Geometry check sheet. Reference: the model listing, model coordinates, mm. Face numbers are marked on the shaded views. A direction names the side the tool comes from. Round coordinates to 2 decimals unless told otherwise and drop trailing zeros. Order: outer loops, then holes, each group sorted by start corner. A loop starts at its lowest first (then second) coordinate and runs counter-clockwise, first axis right, second up.
```python
from build123d import *

# Parameters (mm, degrees)
EXTRUDE_1_DEPTH                 = 206
SKETCH_3_W                      = 252
SKETCH_3_H                      = 252
CUT_EXTRUDE_1_DEPTH             = 123.6
SKETCH_5_W                      = 210
SKETCH_5_H                      = 210
CUT_EXTRUDE_5_DEPTH             = 20.6
SHELL_9_T                       = -5
SKETCH_6_R                      = 50
CUT_EXTRUDE_6_DEPTH             = 455.80065963
RIB_START                       = -5
RIB_1_DEPTH                     = 10
PATTERN_CIRCULAR_1_COUNT        = 4
PATTERN_START                   = -5
PATTERN_CIRCULAR_1_COPY_1_DEPTH = 10
PATTERN_CIRCULAR_1_COPY_2_DEPTH = 10
PATTERN_CIRCULAR_1_COPY_3_DEPTH = 10


# Read off the part's stored shape, not the designer's step: the rib step
with BuildPart() as part:
    # Sketch 1 → Extrude 1 (new body)
    with BuildSketch(Plane(origin=(0, 0, 0), x_dir=(1, 0, 0), z_dir=(0, 1, 0))):
        Polygon((-305, 183), (-183, 305), (183, 305), (305, 183), (305, -183), (183, -305), (-183, -305), (-305, -183), align=None)
    extrude(amount=EXTRUDE_1_DEPTH)

    # Sketch 3 → Cut-Extrude 1 (cut)
    with BuildSketch(Plane(origin=(0, 206, 0), x_dir=(1, 0, 0), z_dir=(0, 1, 0))):
        Rectangle(SKETCH_3_W, SKETCH_3_H)
    extrude(amount=-CUT_EXTRUDE_1_DEPTH, mode=Mode.SUBTRACT)

    # Sketch 5 → Cut-Extrude 5 (cut)
    with BuildSketch(Plane(origin=(0, 82.4, 0), x_dir=(1, 0, 0), z_dir=(0, 1, 0))):
        Rectangle(SKETCH_5_W, SKETCH_5_H)
    extrude(amount=-CUT_EXTRUDE_5_DEPTH, mode=Mode.SUBTRACT)

    # Shell 9
    shell_9_openings = [part.faces().sort_by_distance(p)[0] for p in [
        (0, 0, 0),
    ]]
    offset(amount=SHELL_9_T, openings=shell_9_openings, kind=Kind.INTERSECTION)

    # Sketch 6 → Cut-Extrude 6 (cut, through all)
    with BuildSketch(Plane(origin=(0, 61.8, 0), x_dir=(1, 0, 0), z_dir=(0, 1, 0))):
        with Locations(Location((0, 0, 0), (0, 0, 270))):
            Circle(SKETCH_6_R)
    extrude(amount=-CUT_EXTRUDE_6_DEPTH, mode=Mode.SUBTRACT)

    # Rib 1 outline → Rib 1 (add)
    with BuildSketch(Plane.XY.offset(91.5).offset(RIB_START)):
        Polygon((-300, 112.19925974), (-131, 82.4), (-131, 201), (-300, 201), align=None)
    rib_1 = extrude(amount=RIB_1_DEPTH)

    # Mirror 1: Rib 1 across plane
    add(rib_1.mirror(Plane.XY))

    # Pattern Circular 1: Rib 1 ×4 about axis
    pattern_circular_1_axis = Axis((0, 0, 0), (0, 1, 0))
    for i in range(1, PATTERN_CIRCULAR_1_COUNT):
        add(rib_1.rotate(pattern_circular_1_axis, i * 360 / PATTERN_CIRCULAR_1_COUNT))

    # Pattern Circular 1 copy 1 sketch → Pattern Circular 1 copy 1 (add)
    with BuildSketch(Plane(origin=(-91.5, 0, 0), x_dir=(0, 0, -1), z_dir=(-1, 0, 0)).offset(PATTERN_START)):
        Polygon((-300, -112.19925974), (-131, -82.4), (-131, -201), (-300, -201), align=None)
    extrude(amount=PATTERN_CIRCULAR_1_COPY_1_DEPTH)

    # Pattern Circular 1 copy 2 sketch → Pattern Circular 1 copy 2 (add)
    with BuildSketch(Plane(origin=(0, 0, 91.5), x_dir=(-1, 0, 0), z_dir=(0, 0, 1)).offset(PATTERN_START)):
        Polygon((-300, -112.19925974), (-131, -82.4), (-131, -201), (-300, -201), align=None)
    extrude(amount=PATTERN_CIRCULAR_1_COPY_2_DEPTH)

    # Pattern Circular 1 copy 3 sketch → Pattern Circular 1 copy 3 (add)
    with BuildSketch(Plane(origin=(91.5, 0, 0), x_dir=(0, 0, 1), z_dir=(1, 0, 0)).offset(PATTERN_START)):
        Polygon((-300, -112.19925974), (-131, -82.4), (-131, -201), (-300, -201), align=None)
    extrude(amount=PATTERN_CIRCULAR_1_COPY_3_DEPTH)


solid = part.part
```
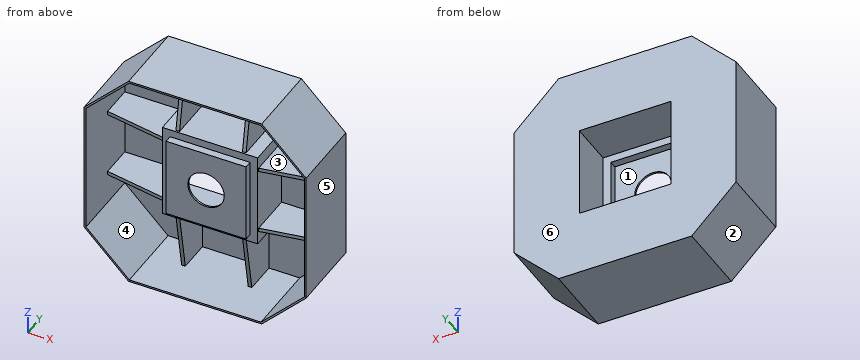
(1) Sectioned sample at A-A, the plane x = 0. Record the cut outline in (y, z), and give its area (3 significant figures).
Returned:
outline: (0, -305) - (206, -305) - (206, -126) - (82.4, -126) - (82.4, -105) - (61.8, -105) - (61.8, -50) - (56.8, -50) - (56.8, -110) - (77.4, -110) - (77.4, -131) - (201, -131) - (201, -300) - (0, -300) - close; (0, 300) - (201, 300) - (201, 131) - (77.4, 131) - (77.4, 110) - (56.8, 110) - (56.8, 50) - (61.8, 50) - (61.8, 105) - (82.4, 105) - (82.4, 126) - (206, 126) - (206, 305) - (0, 305) - close
area: 6,000 mm2
(2) Draft check along X on the marked faces 4, 5 and 6. Enter one of: released by +X, released by -X, zero draft, split by the parting line, or undercut.
Returned:
face 4: undercut
face 5: released by +X
face 6: zero draft
(3) Set-up check for the marked faces 1, 2 and 3: record each of +Z, -Z, +X, -X, +Y, -Y from which the full face is reachable in a straight line by a thin tool's end or side.
Returned:
face 1: +Y
face 2: -Z, -X, +Y, -Y
face 3: -Y
(4) Material ranges on line 1 (X direction, y = 130.5, z = -68); line 2 (X direction, y = 60.75, z = 0); line 3 (Z direction, x = 64.5, y = 57.5), recorded low to high.
Returned:
line 1: x = -305 to -300, -131 to -126, 126 to 131, 300 to 305
line 2: x = -305 to -300, -110 to -50, 50 to 110, 300 to 305
line 3: z = -305 to -300, -110 to 110, 300 to 305
(5) Sectioned sample at D-D, the plane y = 181.5. Give the number of separate pieces and of enclosed holes in the cut face, and give its area (3 significant figures).
Returned:
separate pieces: 1
enclosed holes: 9
area: 29,300 mm2
(6) Sectioned sample at B-B, the plane y = 29. Record the cut outline in (x, z), and give its area (3 significant figures).
Returned:
outline: (-305, -183) - (-183, -305) - (183, -305) - (305, -183) - (305, 183) - (183, 305) - (-183, 305) - (-305, 183) - close; hole (-300, -180.93) - (-180.93, -300) - (180.93, -300) - (300, -180.93) - (300, 180.93) - (180.93, 300) - (-180.93, 300) - (-300, 180.93) - close
area: 10,700 mm2
(7) Depth check by flat-ended pin: P1, Ø5, axis at x = 30.5, z = 112, coming from the +Y side; P2, Ø1, axis at x = -229.5, y = 76, coming from the -Z side; P3, Ø1.5, axis at x = 36, z = -140.5, coming from the -Y side. Enter the tip coordinate at first touch or a pass-through.
Returned:
P1: stops at y = 82.4
P2: stops at z = -259
P3: stops at y = 201
(8) Sectioned sample at C-C, the plane z = 0. Record the cut outline in (x, y).
Returned:
outline: (-305, 0) - (-300, 0) - (-300, 201) - (-131, 201) - (-131, 77.4) - (-110, 77.4) - (-110, 56.8) - (-50, 56.8) - (-50, 61.8) - (-105, 61.8) - (-105, 82.4) - (-126, 82.4) - (-126, 206) - (-305, 206) - close; (50, 56.8) - (110, 56.8) - (110, 77.4) - (131, 77.4) - (131, 201) - (300, 201) - (300, 0) - (305, 0) - (305, 206) - (126, 206) - (126, 82.4) - (105, 82.4) - (105, 61.8) - (50, 61.8) - close
